Design review of the part built by this model. Coordinates are the model's own, in mm. A direction names the side the tool comes from. Round coordinates to 2 decimals unless told otherwise and drop trailing zeros. Loops run counter-clockwise (first coordinate to the right, second up) from the corner with the lowest first, then second, coordinate; pieces in that order, holes last. Notation, with made-up numbers: (-25.75, -13) - (-14.75, -13) arc R32 cw to (-14.75, 15) - close; hole circle Ø7 at (-34.75, 15). An arc over 180 degrees is marked (long way). Return JSON: item names as keys, results as strings. Group by question number.
(1) Wall thickness on L1, parallel to Y at x = 17, z = 56; L2, parallel to X at y = -51, z = 61; L3, parallel to X at y = 28.5, z = 7: over which ranges is each line inside the solid? List them lowest first. Write a range as [from, to].
(2) For faces 1 (the flat face through (-16, -11, 37)), 2 (the flat face through (10, -35, 43)), 3 (the flat face through (22, -22, 32)), 4 (the cylindrical face through (0, 45, 8)), 5 (the flat face through (0, -1, 16)), list the 3-axis set-ups (+Z, -Z, +X, -X, +Y, -Y) from which the entire face can be reached by the end or side of a thin tool; tool diameter is ignored.
(3) The part is to be moulded in two halves that separate along Y. For faces 6 (the flat face through (0, -1, 0)), 7 (the flat face through (16, -11, 37)), 8 (the cylindrical face through (16.08, -37.17, 65.76)), say which applies: pulls with the +Y half, pulls with the -Y half, needs draft (parallel to the pull), parting line crosses it, or undercut.
(4) We need section D-D, the plane z = 8.5. Write out the cut boundary in (x, y), and give its area (3 significant figures).
(5) We need section B-B, the plane z = 19.5. Write out the cut boundary in (x, y), and give its area (3 significant figures).
(6) We need section C-C, the plane y = -35. Write out the cut boundary in (x, z), and give its area (3 significant figures).
(7) We need section A-A, the plane x = 0. Write out the cut boundary in (y, z), and give its area (3 significant figures).
(8) Clearance check with flat-ended pins moving along their axes: pin 1 (3 mm diameter, centred on x = 16, z = 64.5, fed in from +Y); pin 2 (8 mm diameter, centred on x = -4.5, z = 39.5, fed in from -Y); pin 3 (1.5 mm diameter, centred on x = 16, z = 61.5, fed in from +Y); pin 4 (13 mm diameter, centred on x = -18, z = 30.5, fed in from +Y). State where each tip first meets the part, or that it passes through.
from build123d import *

# Parameters (mm, degrees)
ESQUISSE1_R             = 22
BOSS_EXTRU_1_DEPTH      = 16
ENL_V_MAT_EXTRU_1_DEPTH = 16
BOSS_EXTRU_3_DEPTH      = 12
CONG_2_R                = 2


with BuildPart() as part:
    # Esquisse1 → Boss.-Extru.1 (new body)
    with BuildSketch(Plane(origin=(0, 0, 0), x_dir=(0, 1, 0), z_dir=(0, 0, 1))):
        with BuildLine():
            Line((-59, 22), (-59, -22))
            Line((-59, -22), (37, -22))
            ThreePointArc((37, -22), (15, 0), (37, 22))
            Line((37, 22), (-59, 22))
        make_face()
        with Locations((37, 0)):
            Circle(ESQUISSE1_R)
    extrude(amount=BOSS_EXTRU_1_DEPTH)

    # Esquisse2 → Enlèv. mat.-Extru.1 (cut)
    with BuildSketch(Plane(origin=(0, 0, 0), x_dir=(1, 0, 0), z_dir=(0, 0, -1))):
        with BuildLine():
            Line((-8, -37), (-8, -13))
            ThreePointArc((-8, -13), (0, -5), (8, -13))
            Line((8, -13), (8, -37))
            ThreePointArc((8, -37), (0, -45), (-8, -37))
        make_face()
    extrude(amount=-ENL_V_MAT_EXTRU_1_DEPTH, mode=Mode.SUBTRACT)

    # Esquisse3 → Boss.-Extru.3 (add)
    with BuildSketch(Plane.YZ.offset(22)):
        with BuildLine():
            Line((-59, 56), (-59, 16))
            Line((-59, 16), (-11, 16))
            Line((-11, 16), (-11, 56))
            ThreePointArc((-11, 56), (-35, 32), (-59, 56))
        make_face()
        with BuildLine():
            ThreePointArc((-11, 56), (-35, 80), (-59, 56))
            Line((-59, 56), (-45, 56))
            ThreePointArc((-45, 56), (-35, 66), (-25, 56))
            Line((-25, 56), (-11, 56))
        make_face()
        with BuildLine():
            Line((-45, 56), (-59, 56))
            ThreePointArc((-59, 56), (-35, 32), (-11, 56))
            Line((-11, 56), (-25, 56))
            ThreePointArc((-25, 56), (-35, 46), (-45, 56))
        make_face()
    boss_extru_3 = extrude(amount=-BOSS_EXTRU_3_DEPTH)

    # Symétrie1: Boss.-Extru.3 across plane
    add(boss_extru_3.mirror(Plane(origin=(0, 0, 0), x_dir=(0, 0, 1), z_dir=(1, 0, 0))))

    # Congé2
    cong_2_edges = [part.edges().sort_by_distance(p)[0] for p in [
        (16, -11, 16),
        (10, -35, 16),
        (-16, -11, 16),
        (-10, -35, 16),
    ]]
    fillet(cong_2_edges, radius=CONG_2_R)


solid = part.part
Solutions:
{
 "1": {"L1": "[-59, -45], [-25, -11]", "L2": "[-22, -10], [10, 22]", "L3": "[-22, -8], [8, 22]"},
 "2": {"face 1": "+Z, +X, -X, +Y", "face 2": "+Z, +Y, -Y", "face 3": "+Z, -Z, +X, +Y, -Y", "face 4": "+Z, -Z", "face 5": "+Z, +Y"},
 "3": {"face 6": "needs draft", "face 7": "pulls with the +Y half", "face 8": "undercut"},
 "4": {"outline": "(-22, -59) - (22, -59) - (22, 37) arc R22 ccw to (-22, 37) - close; hole (-8, 13) arc R8 ccw to (8, 13) - (8, 37) arc R8 ccw to (-8, 37) - close", "area": "4,400 mm^2"},
 "5": {"outline": "(-22, -59) - (-10, -59) - (-10, -11) - (-22, -11) - close; (10, -59) - (22, -59) - (22, -11) - (10, -11) - close", "area": "1,150 mm^2"},
 "6": {"outline": "(-22, 0) - (22, 0) - (22, 46) - (10, 46) - (10, 18) arc R2 cw to (8, 16) - (-8, 16) arc R2 cw to (-10, 18) - (-10, 46) - (-22, 46) - close; (-22, 66) - (-10, 66) - (-10, 80) - (-22, 80) - close; (10, 66) - (22, 66) - (22, 80) - (10, 80) - close", "area": "1,760 mm^2"},
 "7": {"outline": "(-59, 0) - (5, 0) - (5, 16) - (-59, 16) - close; (45, 0) - (59, 0) - (59, 16) - (45, 16) - close", "area": "1,250 mm^2"},
 "8": {"pin 1": "y = -12.04", "pin 2": "through", "pin 3": "y = -11.47", "pin 4": "y = -11"}
}
